Geometry check sheet. Reference: the model listing, model coordinates, mm. A direction names the side the tool comes from. Give positions to 0.01 mm unless a question says otherwise; leave off trailing zeros. Write each loop counter-clockwise with the first axis right and the second up, starting at its lowest first coordinate (ties: lowest second). Pieces come first, ordered by that corner, then holes. Notation, with made-up numbers: (9.25, 61) - (21.25, 61) arc R8 ccw to (21.25, 68) - close; hole circle Ø4 at (20.5, 69). An arc over 180 degrees is marked (long way). One line per question, with ' | ' between items. Start each with the question number.
Q1. Gauge pin test, flat end, axial feed: P1, Ø10, axis at y = -13.5, z = 38.5, coming from the +X side. Record the tip position at first contact, or that the pin passes through.
Q2. Release check for a two-part mould opening along Z. For faces 1 (the face through (7, 0, -57.15)), 2 (the face through (7, 19.05, 1)), 3 (the face through (7, -25.4, 1)), 4 (the face through (7, 0, 63.5)) record: +Z half, -Z half, draft (parallel to the pull), parting line (faces both ways), or undercut.
Q3. Set-up check for faces 5 (the face through (7, 0, 57.15)), 6 (the face through (7, 25.4, -1)): record each of +Z, -Z, +X, -X, +Y, -Y from which the full face is reachable in a straight line by a thin tool's end or side.
Q4. Section check C-C on y = 0.5. Record the boundary of the cut face in (x, z).
Q5. Section check B-B on x = -245. Record the boundary of the cut face in (y, z).
Q6. Section check A-A on z = -5.5. Record the boundary of the cut face in (x, y), and give its area (3 significant figures).
Q7. Thickness scan on L1, parallel to Y at x = -331.5, z = -5; L2, parallel to Z at x = -55, y = 12; L3, parallel to Z at x = 199, y = 13.5. Record the ranges inside material, lowest first. Write a range as [from, to].
```python
from build123d import *

# Parameters (mm, degrees)
F3_DEPTH = 500


with BuildPart() as f3:
    # F2 (on Right) → F3 (new body, symmetric)
    with BuildSketch(Plane.YZ):
        with BuildLine():
            ThreePointArc((25.4, 50.8), (21.680256, 59.780256), (12.7, 63.5))
            Line((12.7, 63.5), (-12.7, 63.5))
            ThreePointArc((-12.7, 63.5), (-21.680256, 59.780256), (-25.4, 50.8))
            Line((-25.4, 50.8), (-25.4, -50.8))
            ThreePointArc((-25.4, -50.8), (-21.680256, -59.780256), (-12.7, -63.5))
            Line((-12.7, -63.5), (12.7, -63.5))
            ThreePointArc((12.7, -63.5), (21.680256, -59.780256), (25.4, -50.8))
            Line((25.4, -50.8), (25.4, 50.8))
        make_face()
        with BuildLine():
            Line((-12.7, 57.15), (12.7, 57.15))
            ThreePointArc((12.7, 57.15), (17.190128, 55.290128), (19.05, 50.8))
            Line((19.05, 50.8), (19.05, -50.8))
            ThreePointArc((19.05, -50.8), (17.190128, -55.290128), (12.7, -57.15))
            Line((12.7, -57.15), (-12.7, -57.15))
            ThreePointArc((-12.7, -57.15), (-17.190128, -55.290128), (-19.05, -50.8))
            Line((-19.05, -50.8), (-19.05, 50.8))
            ThreePointArc((-19.05, 50.8), (-17.190128, 55.290128), (-12.7, 57.15))
        make_face(mode=Mode.SUBTRACT)
    extrude(amount=F3_DEPTH, both=True)


with BuildPart() as f0_1:
    # F0: copy of F3
    add(f3.part)


solid = f3.part
```
Working result:
1) P1: passes through
2) face 1: undercut | face 2: undercut | face 3: draft | face 4: +Z half
3) face 5: +X, -X | face 6: +Z, -Z, +X, -X, +Y
4) outline: (-500, -63.5) - (500, -63.5) - (500, -57.15) - (-500, -57.15) - close; (-500, 57.15) - (500, 57.15) - (500, 63.5) - (-500, 63.5) - close
5) outline: (-25.4, -50.8) arc R12.7 ccw to (-12.7, -63.5) - (12.7, -63.5) arc R12.7 ccw to (25.4, -50.8) - (25.4, 50.8) arc R12.7 ccw to (12.7, 63.5) - (-12.7, 63.5) arc R12.7 ccw to (-25.4, 50.8) - close; hole (-19.05, -50.8) arc R6.35 ccw to (-12.7, -57.15) - (12.7, -57.15) arc R6.35 ccw to (19.05, -50.8) - (19.05, 50.8) arc R6.35 ccw to (12.7, 57.15) - (-12.7, 57.15) arc R6.35 ccw to (-19.05, 50.8) - close
6) outline: (-500, -25.4) - (500, -25.4) - (500, -19.05) - (-500, -19.05) - close; (-500, 19.05) - (500, 19.05) - (500, 25.4) - (-500, 25.4) - close | area: 12,700 mm2
7) L1: y = [-25.4, -19.05], [19.05, 25.4] | L2: z = [-63.5, -57.15], [57.15, 63.5] | L3: z = [-63.47, -57.1], [57.1, 63.47]
